Read the model definition and answer for the solid it produces. Units are mm, in the model's axes. Round coordinates to 2 decimals unless told otherwise and drop trailing zeros. Write each loop counter-clockwise with the first axis right and the second up, starting at its lowest first coordinate (ties: lowest second). Pieces come first, ordered by that corner, then holes. Notation, with made-up numbers: (-28, 59.5) - (-9, 59.5) arc R32 cw to (-9, 88.5) - close; hole circle Ø9 at (25, 5). An arc over 180 degrees is marked (long way). One line per item, written item: value. Start each with the question number.
(1) A flat-ended cylindrical pin translates along its axis: pin 1 Ø1 at (y, z) = (2.5, 124.5) entering from -X. Find the tip coordinate at first contact, or state that the pin passes through.
(2) A cutting plane is placed at B-B, the plane z = 121.5. Determine the outline of the cut face in (x, y).
(3) A cutting plane is placed at A-A, the plane y = 2.6. Determine the outline of the cut face in (x, z).
(4) Find the intervals of material crossed by L1, parallel to X at y = 4.35, z = 118.5, in increasing order.
(5) The mould has two halves that part along Z. Classify faces 1 (the face through (137, 2, 53)), 2 (the face through (13.497, 2.465, 121.203)), 3 (the face through (68, 2, 0)): +Z half, -Z half, draft (parallel to the pull), parting line (faces both ways), or undercut.
Autodesk Inventor part; units mm, degrees
ref_plane "YZ Plane" through (0, 0, 0) normal (1, 0, 0) x (0, 1, 0)
ref_plane "XZ Plane" through (0, 0, 0) normal (0, 1, 0) x (-1, 0, 0)
ref_plane "XY Plane" through (0, 0, 0) normal (0, 0, 1) x (1, 0, 0)
sketch "Sketch2" plane through (0, 0, 0) normal (0, 1, 0) x (-1, 0, 0)
  line L0 (0, 0) -> (-137, 0)
  line L1 (-137, 144) -> (0, 144)
  line L2 (0, 144) -> (-137, 144)
  line L3 (-137, 144) -> (-137, 134.2279)
  line L4 (0, 135) -> (0, 144)
  arc A0 (0, 135) -> (0, 108) centre (0, 121.5) ccw
  line L5 (-137, 0) -> (-137, 108.7721)
  line L6 (-137, 134.2279) -> (-137, 144)
  line L7 (0, 144) -> (0, 135)
  line L8 (0, 108) -> (0, 0)
  arc A1 (-137, 108) -> (-137, 135) centre (-137, 121.5) ccw
  point P0 (-13.5, 121.5)
  point P1 (-123.5, 121.5)
  dimension "d0" = 137
  dimension "d4" = 27
  dimension "d6" = 27
  dimension "d7" = 110
  dimension "d8" = 22.5
extrude "Extrusion1" add sketch "Sketch2" along normal blind 5
properties part number "Cover"
Here are the results:
1. pin 1: x = 13.04
2. outline: (13.5, 0) - (123.5, 0) - (123.5, 5) - (13.5, 5) - close
3. outline: (0, 0) - (137, 0) - (137, 108) arc R13.5 cw to (137, 135) - (137, 144) - (0, 144) - (0, 135) arc R13.5 cw to (0, 108) - close
4. L1: 13.16 to 123.84
5. face 1: draft
5. face 2: undercut
5. face 3: -Z half
